Geometry: final body of the model. Coordinates: model frame, mm. A direction names the side the tool comes from. Round coordinates to 2 decimals unless told otherwise and drop trailing zeros. Loops run counter-clockwise (first coordinate to the right, second up) from the corner with the lowest first, then second, coordinate; pieces in that order, holes last. Notation, with made-up numbers: (-21.5, -30) - (-12.5, -30) arc R20 cw to (-12.5, 9) - close; hole circle Ø11 at (66.25, 47). An arc over 180 degrees is marked (long way). Write item = value, one per line. Start each with the question number.
Item 1: Section A-A (x = 97). Return loops of the section in (y, z), plus the area to 3 significant figures.
Item 2: Section C-C (y = 14.5). Count the separate pieces of the cut face and the enclosed holes in it, plus the area to 3 significant figures.
Item 3: Access query for faces 4 (the cylindrical face through (82.96, 3.203, 1.479)), 5 (the flat face through (117, 25, 30)), 6 (the flat face through (59, 0, 35)), 7 (the flat face through (70.797, 25, 1)). Directions: +Z, -Z, +X, -X, +Y, -Y. A direction counts if a zero-diameter tool reaches every point of the face in a straight line with its end or side. Return the directions, or none.
Item 4: Section D-D (x = 44). Return loops of the section in (y, z).
Item 5: Line query: line 1 (X direction, y = 5, z = 5.75); line 2 (X direction, y = 19, z = 55.5); line 3 (Y direction, x = 7, z = 26.5). Output: solid intervals per line, ascending. Write a range as from..to.
Item 6: Section B-B (z = 31.5). Return loops of the section in (x, y).
Item 7: First-contact query: pin 1 (1.5 mm diameter, centred on x = 56.5, z = 57, fed in from +Y); pin 2 (7 mm diameter, centred on x = 34.5, y = 44.5, fed in from +Z); pin 3 (12 mm diameter, centred on x = 34.5, z = 51.5, fed in from +Y). Flat tips, straight axial feed; report the tip coordinate or a pass-through.
Item 8: Draft query along Z for faces 1 (the flat face through (58.67, 41.37, 48.39)), 2 (the cylindrical face through (68.96, 3.203, 1.479)), 3 (the flat face through (59, 48, 22)). Return one class per face: pulls with the +Z half, pulls with the -Z half, needs draft (parallel to the pull), parting line crosses it, or undercut.
from build123d import *

# Parameters (mm, degrees)
SKETCH1_W               = 119
SKETCH1_H               = 50
BOSS_EXTRUDE1_DEPTH     = 70
SKETCH2_W               = 115
SKETCH2_H               = 46
CUT_EXTRUDE1_DEPTH      = 67
SKETCH3_W               = 50
SKETCH3_H               = 29
CUT_EXTRUDE2_DEPTH      = 10
SKETCH4_R               = 1.95
CUT_EXTRUDE3_DEPTH      = 10
SKETCH5_R               = 3.25
SKETCH5_R_2             = 1.95
BOSS_EXTRUDE3_DEPTH     = 10
FILLET1_R               = 2
SKETCH6_R               = 2
CUT_EXTRUDE4_DEPTH      = 10
CUT_EXTRUDE5_DEPTH      = 146.220522014
CUT_EXTRUDE5_DEPTH_BACK = 146.220522014
SKETCH8_R               = 2
BOSS_EXTRUDE4_DEPTH     = 115
CUT_EXTRUDE6_DEPTH      = 146.220522014
CUT_EXTRUDE6_DEPTH_BACK = 146.220522014
FILLET2_R               = 14
CUT_EXTRUDE8_DEPTH      = 10
CUT_EXTRUDE9_DEPTH      = 143.341139563


with BuildPart() as part:
    # Sketch1 → Boss-Extrude1 (new body)
    with BuildSketch(Plane.XY):
        with Locations((59.5, 25)):
            Rectangle(SKETCH1_W, SKETCH1_H)
    extrude(amount=BOSS_EXTRUDE1_DEPTH)

    # Sketch2 → Cut-Extrude1 (cut)
    with BuildSketch(Plane.XY.offset(70)):
        with Locations((59.5, 25)):
            Rectangle(SKETCH2_W, SKETCH2_H)
    extrude(amount=-CUT_EXTRUDE1_DEPTH, mode=Mode.SUBTRACT)

    # Sketch3 → Cut-Extrude2 (cut)
    with BuildSketch(Plane.XY.offset(3)):
        with Locations((33, 25)):
            Rectangle(SKETCH3_W, SKETCH3_H)
    extrude(amount=-CUT_EXTRUDE2_DEPTH, mode=Mode.SUBTRACT)

    # Sketch4 → Cut-Extrude3 (cut)
    with BuildSketch(Plane(origin=(0, 0, 0), x_dir=(-1, 0, 0), z_dir=(0, 0, -1))):
        with Locations((-32.95, 45)):
            Circle(SKETCH4_R)
        with Locations((-32.95, 5)):
            Circle(SKETCH4_R)
    extrude(amount=-CUT_EXTRUDE3_DEPTH, mode=Mode.SUBTRACT)

    # Sketch5 → Boss-Extrude3 (add)
    # profile 1 of 2: a face of its own
    with BuildSketch(Plane.XY.offset(3)):
        with Locations((32.95, 45)):
            Circle(SKETCH5_R)
        with Locations(Location((32.95, 45, 0), (0, 0, 180))):
            Circle(SKETCH5_R_2, mode=Mode.SUBTRACT)
    # profile 2 of 2: a face of its own
    with BuildSketch(Plane.XY.offset(3)):
        with Locations((32.95, 5)):
            Circle(SKETCH5_R)
        with Locations(Location((32.95, 5, 0), (0, 0, 180))):
            Circle(SKETCH5_R_2, mode=Mode.SUBTRACT)
    extrude(amount=BOSS_EXTRUDE3_DEPTH)

    # Fillet1
    fillet1_edges = [part.edges().sort_by_distance(p)[0] for p in [
        (31.147224362, 42.295836543, 3),
        (31.147224362, 7.704163457, 3),
    ]]
    fillet(fillet1_edges, radius=FILLET1_R)

    # Sketch6 → Cut-Extrude4 (cut)
    with BuildSketch(Plane(origin=(0, 2, 0), x_dir=(1, 0, 0), z_dir=(0, 1, 0))):
        with Locations(Location((85, -65.5, 0), (0, 0, 180))):
            Circle(SKETCH6_R)
        with Locations(Location((35, -65.5, 0), (0, 0, 180))):
            Circle(SKETCH6_R)
    extrude(amount=-CUT_EXTRUDE4_DEPTH, mode=Mode.SUBTRACT)

    # Sketch8 → Cut-Extrude5 (cut, two sides: drawn at the far end of the back side and taken through both)
    with BuildSketch(Plane(origin=(2, 0, 0), x_dir=(0, 0, -1), z_dir=(1, 0, 0)).offset(-CUT_EXTRUDE5_DEPTH_BACK)):
        with Locations(Location((-65.5, 14.5, 0), (0, 0, 90))):
            Circle(SKETCH8_R)
    extrude(amount=CUT_EXTRUDE5_DEPTH + CUT_EXTRUDE5_DEPTH_BACK, mode=Mode.SUBTRACT)

    # Sketch9 → Boss-Extrude4 (add)
    with BuildSketch(Plane(origin=(2, 0, 0), x_dir=(0, 0, -1), z_dir=(1, 0, 0))):
        Polygon((-55.594060536, 32.500624229), (-43.169621176, 48), (-41.169621176, 48), (-53.594060926, 32.499375771), align=None)
    extrude(amount=BOSS_EXTRUDE4_DEPTH)

    # Sketch10 → Cut-Extrude6 (cut, two sides: drawn at the far end of the back side and taken through both)
    with BuildSketch(Plane(origin=(2, 0, 0), x_dir=(0, 0, -1), z_dir=(1, 0, 0)).offset(-CUT_EXTRUDE6_DEPTH_BACK)):
        Polygon((-55.471753528, 32.500624229), (-70, 32.500624229), (-70, 50), (-41.5, 50), align=None)
    extrude(amount=CUT_EXTRUDE6_DEPTH + CUT_EXTRUDE6_DEPTH_BACK, mode=Mode.SUBTRACT)

    # Fillet2
    fillet2_edges = [part.edges().sort_by_distance(p)[0] for p in [
        (118, 32.500624229, 70),
        (1, 32.500624229, 70),
    ]]
    fillet(fillet2_edges, radius=FILLET2_R)

    # Sketch11 → Cut-Extrude8 (cut)
    with BuildSketch(Plane(origin=(0, 0, 0), x_dir=(-1, 0, 0), z_dir=(0, 0, -1))):
        with BuildLine():
            Line((-109.202811856, 45), (-109.202811856, 5))
            ThreePointArc((-109.202811856, 5), (-111, 3.202811856), (-112.797188144, 5))
            Line((-112.797188144, 5), (-112.797188144, 45))
            ThreePointArc((-112.797188144, 45), (-111, 46.797188144), (-109.202811856, 45))
        make_face()
        with BuildLine():
            Line((-102.202811856, 45), (-102.202811856, 5))
            ThreePointArc((-102.202811856, 5), (-104, 3.202811856), (-105.797188144, 5))
            Line((-105.797188144, 5), (-105.797188144, 45))
            ThreePointArc((-105.797188144, 45), (-104, 46.797188144), (-102.202811856, 45))
        make_face()
        with BuildLine():
            Line((-95.202811856, 45), (-95.202811856, 5))
            ThreePointArc((-95.202811856, 5), (-97, 3.202811856), (-98.797188144, 5))
            Line((-98.797188144, 5), (-98.797188144, 45))
            ThreePointArc((-98.797188144, 45), (-97, 46.797188144), (-95.202811856, 45))
        make_face()
        with BuildLine():
            Line((-88.202811856, 45), (-88.202811856, 5))
            ThreePointArc((-88.202811856, 5), (-90, 3.202811856), (-91.797188144, 5))
            Line((-91.797188144, 5), (-91.797188144, 45))
            ThreePointArc((-91.797188144, 45), (-90, 46.797188144), (-88.202811856, 45))
        make_face()
        with BuildLine():
            Line((-81.202811856, 45), (-81.202811856, 5))
            ThreePointArc((-81.202811856, 5), (-83, 3.202811856), (-84.797188144, 5))
            Line((-84.797188144, 5), (-84.797188144, 45))
            ThreePointArc((-84.797188144, 45), (-83, 46.797188144), (-81.202811856, 45))
        make_face()
        with BuildLine():
            Line((-74.202811856, 45), (-74.202811856, 5))
            ThreePointArc((-74.202811856, 5), (-76, 3.202811856), (-77.797188144, 5))
            Line((-77.797188144, 5), (-77.797188144, 45))
            ThreePointArc((-77.797188144, 45), (-76, 46.797188144), (-74.202811856, 45))
        make_face()
        with BuildLine():
            Line((-67.202811856, 45), (-67.202811856, 5))
            ThreePointArc((-67.202811856, 5), (-69, 3.202811856), (-70.797188144, 5))
            Line((-70.797188144, 5), (-70.797188144, 45))
            ThreePointArc((-70.797188144, 45), (-69, 46.797188144), (-67.202811856, 45))
        make_face()
    extrude(amount=-CUT_EXTRUDE8_DEPTH, mode=Mode.SUBTRACT)

    # Sketch12 → Cut-Extrude9 (cut, through all)
    with BuildSketch(Plane.XY.offset(10)):
        with BuildLine():
            Line((108.667383108, 28.499375771), (91.910743178, 28.499375771))
            ThreePointArc((91.910743178, 28.499375771), (87.910743178, 32.499375771), (91.910743178, 36.499375771))
            Line((91.910743178, 36.499375771), (108.667383108, 36.499375771))
            ThreePointArc((108.667383108, 36.499375771), (112.667383108, 32.499375771), (108.667383108, 28.499375771))
        make_face()
    extrude(amount=CUT_EXTRUDE9_DEPTH, mode=Mode.SUBTRACT)


solid = part.part
Taken from the geometry:
q1.outline = (0, 0) - (3.2, 0) - (3.2, 3) - (2, 3) - (2, 70) - (0, 70) - close; (36.5, 50.39) - (48, 41.17) - (48, 3) - (46.8, 3) - (46.8, 0) - (50, 0) - (50, 41.5) - (36.5, 52.28) - close
q1.area = 254 mm^2
q2.separate_pieces = 11
q2.enclosed_holes = 0
q2.area = 384 mm^2
q3.face_4 = +Z, -Z
q3.face_5 = none
q3.face_6 = +Z, -Z, +X, -X, -Y
q3.face_7 = -Z
q4.outline = (0, 0) - (10.5, 0) - (10.5, 3) - (2, 3) - (2, 70) - (0, 70) - close; (32.5, 53.59) - (48, 41.17) - (48, 3) - (39.5, 3) - (39.5, 0) - (50, 0) - (50, 41.5) - (32.5, 55.47) - (32.5, 55.59) - close
q5.line_1 = 0..2, 29.7..31, 34.9..36.2, 117..119
q5.line_2 = 0..2, 117..119
q5.line_3 = 0..2, 48..50
q6.outline = (0, 0) - (119, 0) - (119, 50) - (0, 50) - close; hole (2, 2) - (117, 2) - (117, 48) - (2, 48) - close
q7.pin_1 = 2
q7.pin_2 = 48.69
q7.pin_3 = 44.99
q8.face_1 = pulls with the +Z half
q8.face_2 = needs draft
q8.face_3 = undercut
